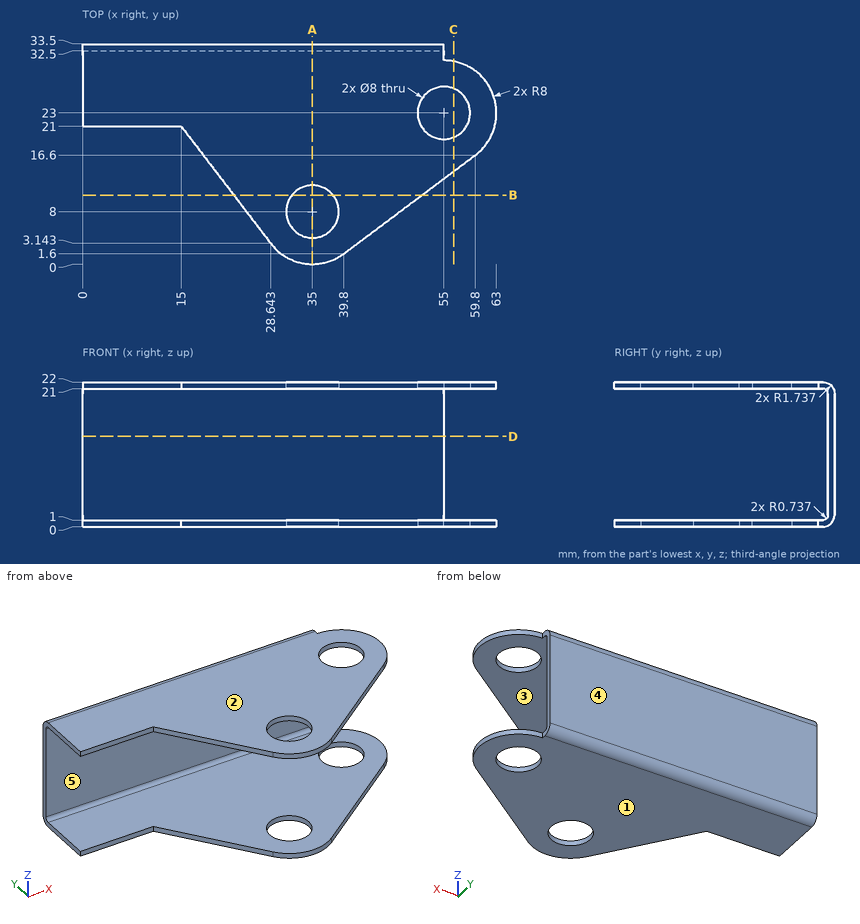
Verification items for this drawing (mm, ordinates from the low corner). A direction names the side the tool comes from. Round coordinates to 2 decimals unless told otherwise and drop trailing zeros. Loops run counter-clockwise (first coordinate to the right, second up) from the corner with the lowest first, then second, coordinate; pieces in that order, holes last. Notation, with made-up numbers: (-19.5, 30) - (-8.5, 30) arc R15 ccw to (-8.5, 51) - close; hole circle Ø3 at (-4.5, 51). An arc over 180 degrees is marked (long way). Write item = value, one per line.
Q1. Depth check by flat-ended pin: pin 1 (5 mm diameter, centred on x = 55, y = 23, fed in from -Z); pin 2 (4 mm diameter, centred on x = 34, z = 13.5, fed in from -Y); pin 3 (2 mm diameter, centred on y = 32.5, z = 15, fed in from +X); pin 4 (0.8 mm diameter, centred on x = 7, z = 0.5, fed in from -Y). Enter the tip coordinate at first touch or a pass-through.
Here are the results:
pin_1 = through
pin_2 = 32.5
pin_3 = 55
pin_4 = 21
Q2. Sectioned sample at A-A on x = 35. Record the boundary of the cut face in (y, z).
Here are the results:
outline = (0, 0) - (4, 0) - (4, 1) - (0, 1) - close; (0, 21) - (4, 21) - (4, 22) - (0, 22) - close; (12, 0) - (31.76, 0) arc R1.74 ccw to (33.5, 1.74) - (33.5, 20.26) arc R1.74 ccw to (31.76, 22) - (12, 22) - (12, 21) - (31.76, 21) arc R0.74 cw to (32.5, 20.26) - (32.5, 1.74) arc R0.74 cw to (31.76, 1) - (12, 1) - close
Q3. Tool access check on the marked faces 4 and 5. Record the directions out of +Z, -Z, +X, -X, +Y, -Y that give a thin tool (end or side, any length) a straight path to the whole face; none if there is none.
Here are the results:
face_4 = +Z, -Z, +X, -X, +Y
face_5 = +X, -X, -Y
Q4. Sectioned sample at C-C on x = 56.5. Record the boundary of the cut face in (y, z) (1 decimal).
Here are the results:
outline = (14.1, 0) - (19.3, 0) - (19.3, 1) - (14.1, 1) - close; (14.1, 21) - (19.3, 21) - (19.3, 22) - (14.1, 22) - close; (26.7, 0) - (30.9, 0) - (30.9, 1) - (26.7, 1) - close; (26.7, 21) - (30.9, 21) - (30.9, 22) - (26.7, 22) - close
Q5. Sectioned sample at D-D on z = 13.75. Record the boundary of the cut face in (x, y).
Here are the results:
outline = (0, 32.5) - (55, 32.5) - (55, 33.5) - (0, 33.5) - close
Q6. Mould release check, pull along Z, two halves, no side actions. Record for the marked faces 1, 2 and 3: +Z half, -Z half, draft (parallel to the pull), parting line (faces both ways), or undercut.
Here are the results:
face_1 = -Z half
face_2 = +Z half
face_3 = undercut
Q7. Sectioned sample at B-B on y = 10.5. Record the boundary of the cut face in (x, z).
Here are the results:
outline = (23.02, 0) - (31.88, 0) - (31.88, 1) - (23.02, 1) - close; (23.02, 21) - (31.88, 21) - (31.88, 22) - (23.02, 22) - close; (38.12, 0) - (51.67, 0) - (51.67, 1) - (38.12, 1) - close; (38.12, 21) - (51.67, 21) - (51.67, 22) - (38.12, 22) - close
Q8. Material ranges on L1, parallel to Z at x = 15, y = 22.5; L2, parallel to Y at x = 45, z = 8.5; L3, parallel to X at y = 8, z = 21.6 (1 decimal), recorded low to high.
Here are the results:
L1 = 0 to 1, 21 to 22
L2 = 32.5 to 33.5
L3 = 24.9 to 31, 39 to 48.3
